Geometry: final body of the model. Coordinates: model frame, mm. Face numbers are marked on the shaded views. Round coordinates to 2 decimals unless told otherwise and drop trailing zeros. Order: outer loops, then holes, each group sorted by start corner. A loop starts at its lowest first (then second) coordinate and runs counter-clockwise, first axis right, second up. Notation, with made-up numbers: (-25.5, 3) -> (-19.5, 3) arc R30 cw to (-19.5, 37) -> close; hole circle Ø10 at (2, -21.5). An arc over 180 degrees is marked (long way). Put each result on its own line as item: value.
```python
from build123d import *

# Parameters (mm, degrees)
SKETCH_1_W      = 41
SKETCH_1_H      = 10
SKETCH_1_R      = 2
EXTRUDE_1_DEPTH = 20
SKETCH_2_W      = 41
SKETCH_2_H      = 3
EXTRUDE_2_DEPTH = 20


with BuildPart() as part:
    # 草图1 → 凸台-拉伸1 (new body)
    with BuildSketch(Plane.XY):
        Rectangle(SKETCH_1_W, SKETCH_1_H)
        with Locations((12.5, 0)):
            Circle(SKETCH_1_R, mode=Mode.SUBTRACT)
        with Locations(Location((-12.5, 0, 0), (0, 0, 180))):
            Circle(SKETCH_1_R, mode=Mode.SUBTRACT)
    extrude(amount=EXTRUDE_1_DEPTH)

    # 草图2 → 凸台-拉伸2 (add)
    with BuildSketch(Plane.XY.offset(20)):
        with Locations((0, -6.5)):
            Rectangle(SKETCH_2_W, SKETCH_2_H)
    extrude(amount=-EXTRUDE_2_DEPTH)


solid = part.part
```
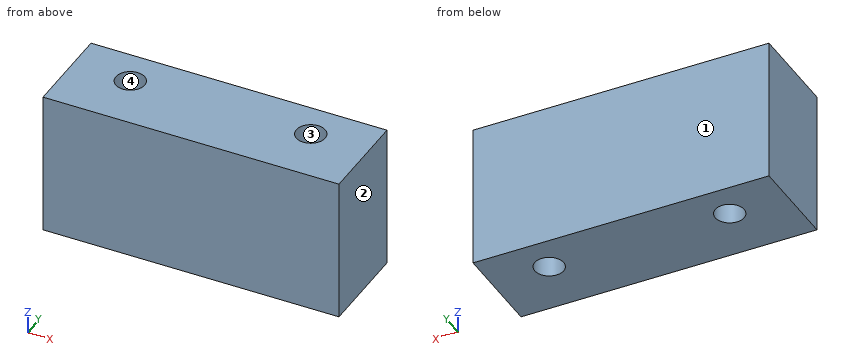
1. Draft query along Y for the marked faces 1, 2, 3 and 4. Return one class per face: +Y half, -Y half, draft (parallel to the pull), parting line (faces both ways), or undercut.
Ans:
face 1: +Y half
face 2: draft
face 3: undercut
face 4: undercut
2. Material intervals for probe 1 along Y at (x, z) = (-12.5, 7.5); probe 2 along X at (y, z) = (-1.5, 2), sorted ascending.
Ans:
probe 1: -8 to -2, 2 to 5
probe 2: -20.5 to -13.82, -11.18 to 11.18, 13.82 to 20.5
3. Cut plane C-C on z = 16.5. Return loops of the section in (x, y), and give its area (3 significant figures).
Ans:
outline: (-20.5, -8) -> (20.5, -8) -> (20.5, 5) -> (-20.5, 5) -> close; hole circle Ø4 at (-12.5, 0); hole circle Ø4 at (12.5, 0)
area: 508 mm²
4. Contact query for flat-ended pins moving along their axis: P1, Ø3, axis at x = -12.5, y = 0, coming from the +Z side; P2, Ø5, axis at x = 12.5, y = 0, coming from the -Z side. Output: stop coordinate, or through.
Ans:
P1: through
P2: z = 0
5. Cut plane A-A on x = -12.5. Return loops of the section in (y, z), and give its area (3 significant figures).
Ans:
outline: (-8, 0) -> (-2, 0) -> (-2, 20) -> (-8, 20) -> close; (2, 0) -> (5, 0) -> (5, 20) -> (2, 20) -> close
area: 180 mm²
6. Cut plane B-B on y = 0. Return loops of the section in (x, z).
Ans:
outline: (-20.5, 0) -> (-14.5, 0) -> (-14.5, 20) -> (-20.5, 20) -> close; (-10.5, 0) -> (10.5, 0) -> (10.5, 20) -> (-10.5, 20) -> close; (14.5, 0) -> (20.5, 0) -> (20.5, 20) -> (14.5, 20) -> close
